Geometry check sheet. Reference: the model listing, model coordinates, mm. A direction names the side the tool comes from. Coordinates: 2 decimals unless noted, no trailing zeros. Write each loop counter-clockwise with the first axis right and the second up, starting at its lowest first coordinate (ties: lowest second). Pieces come first, ordered by that corner, then holes. Notation, with made-up numbers: (86, -15) -> (111, -15) arc R21 ccw to (111, -4) -> close; hole circle Ø3 at (76, 22.25). An arc over 180 degrees is marked (long way). Answer in a Markdown table with one row per item. Add a question column.
1. Set-up check for faces 1 (the flat face through (-38.1, 44, 71)), 2 (the flat face through (-45, 38.1, 71)), 3 (the flat face through (-1, -50.8, 30)): record each of +Z, -Z, +X, -X, +Y, -Y from which the full face is reachable in a straight line by a thin tool's end or side.
2. Cross-section at C-C on z = 49. Record the cut outline in (x, y), and give its area (3 significant figures).
3. Cross-section at A-A on y = 44. Record the cut outline in (x, z), and give its area (3 significant figures).
4. Cross-section at D-D on x = -31.5. Record the cut outline in (y, z).
5. Depth check by flat-ended pin: P1, Ø1, axis at x = -31.5, y = -3, coming from the +Z side; P2, Ø10, axis at x = -15, y = 34.5, coming from the +Z side; P3, Ø1.5, axis at x = 36, z = 87.5, coming from the +Y side; P4, Ø5, axis at x = -5.5, y = 11, coming from the +Z side. Enter the tip coordinate at first touch or a pass-through.
6. Cross-section at B-B on x = -44. Record the cut outline in (y, z), and give its area (3 significant figures).
7. Mould release check, pull along X, two halves, no side actions. Record for faces 4 (the flat face through (50.8, -1, 17)), 5 (the flat face through (-1, 50.8, 30)), 6 (the flat face through (38.1, 44, 71)): pulls with the +X half, pulls with the -X half, needs draft (parallel to the pull), parting line crosses it, or undercut.
8. Scan lines: L1, parallel to X at y = 47, z = 46; L2, parallel to Z at x = 26, y = -42; L3, parallel to Z at x = -30.5, y = -0.5. Record each from-to range of solid material in increasing order. Write a range as from..to.
```python
from build123d import *

# Parameters (mm, degrees)
F0_W     = 101.6
F0_H     = 101.6
F1_DEPTH = 33.02
F2_W     = 12.7
F2_H     = 12.7
F3_DEPTH = 76.2
F4_W     = 101.6
F4_H     = 25.4
F5_DEPTH = 12.7
F6_R     = 5.08


with BuildPart() as f1:
    # F0 (on Top) → F1 (new body)
    with BuildSketch(Plane.XY):
        Rectangle(F0_W, F0_H)
    extrude(amount=F1_DEPTH)

    # F2 (on face) → F3 (join)
    with BuildSketch(Plane.XY.offset(33.02)):
        with Locations((44.45, -44.45)):
            Rectangle(F2_W, F2_H)
        with Locations((-44.45, -44.45)):
            Rectangle(F2_W, F2_H)
        with Locations((-44.45, 44.45)):
            Rectangle(F2_W, F2_H)
        with Locations((44.45, 44.45)):
            Rectangle(F2_W, F2_H)
    extrude(amount=F3_DEPTH)

    # F4 (on face) → F5 (cut)
    with BuildSketch(Plane.XY.offset(33.02)):
        Rectangle(F4_W, F4_H)
    extrude(amount=-F5_DEPTH, mode=Mode.SUBTRACT)

    # F6
    f6_edges = [f1.edges().sort_by_distance(p)[0] for p in [
        (0, 12.7, 33.02),
        (0, -12.7, 33.02),
    ]]
    fillet(f6_edges, radius=F6_R)


solid = f1.part
```
Results found:
| question | item | result |
|---|---|---|
| 1 | face 1 | +Z, +Y, -Y |
| 1 | face 2 | +Z, +X, -X |
| 1 | face 3 | +Z, -Z, +X, -X, -Y |
| 2 | outline | (-50.8, -50.8) -> (-38.1, -50.8) -> (-38.1, -38.1) -> (-50.8, -38.1) -> close; (-50.8, 38.1) -> (-38.1, 38.1) -> (-38.1, 50.8) -> (-50.8, 50.8) -> close; (38.1, -50.8) -> (50.8, -50.8) -> (50.8, -38.1) -> (38.1, -38.1) -> close; (38.1, 38.1) -> (50.8, 38.1) -> (50.8, 50.8) -> (38.1, 50.8) -> close |
| 2 | area | 645 mm^2 |
| 3 | outline | (-50.8, 0) -> (50.8, 0) -> (50.8, 109.22) -> (38.1, 109.22) -> (38.1, 33.02) -> (-38.1, 33.02) -> (-38.1, 109.22) -> (-50.8, 109.22) -> close |
| 3 | area | 5,290 mm^2 |
| 4 | outline | (-50.8, 0) -> (50.8, 0) -> (50.8, 33.02) -> (17.78, 33.02) arc R5.08 ccw to (12.7, 27.94) -> (12.7, 20.32) -> (-12.7, 20.32) -> (-12.7, 27.94) arc R5.08 ccw to (-17.78, 33.02) -> (-50.8, 33.02) -> close |
| 5 | P1 | stops at z = 20.32 |
| 5 | P2 | stops at z = 33.02 |
| 5 | P3 | passes through |
| 5 | P4 | stops at z = 30.68 |
| 6 | outline | (-50.8, 0) -> (50.8, 0) -> (50.8, 109.22) -> (38.1, 109.22) -> (38.1, 33.02) -> (17.78, 33.02) arc R5.08 ccw to (12.7, 27.94) -> (12.7, 20.32) -> (-12.7, 20.32) -> (-12.7, 27.94) arc R5.08 ccw to (-17.78, 33.02) -> (-38.1, 33.02) -> (-38.1, 109.22) -> (-50.8, 109.22) -> close |
| 6 | area | 4,960 mm^2 |
| 7 | face 4 | pulls with the +X half |
| 7 | face 5 | needs draft |
| 7 | face 6 | undercut |
| 8 | L1 | x = -50.8..-38.1, 38.1..50.8 |
| 8 | L2 | z = 0..33.02 |
| 8 | L3 | z = 0..20.32 |
